Can you work these out from the model? Positions are in its coordinate system, mm. A direction names the side the tool comes from. Give positions to 0.01 mm unless a question says otherwise; leave off trailing zeros. Write each loop counter-clockwise with the first axis right and the second up, starting at its lowest first coordinate (ties: lowest second). Pieces come first, ordered by that corner, then holes.
from build123d import *

# Parameters (mm, degrees)
F1_DEPTH = 25.4


with BuildPart() as f1:
    # F0 (on Front) → F1 (new body)
    with BuildSketch(Plane.XZ):
        with BuildLine():
            Line((-1.5875, 51.919649), (-1.5875, 53.951649))
            ThreePointArc((-1.5875, 53.951649), (-9.37266, 53.154998), (-16.960789, 51.240924))
            Line((-16.960789, 51.240924), (-16.265804, 49.331468))
            Line((-16.265804, 49.331468), (-19.249328, 48.245554))
            Line((-19.249328, 48.245554), (-19.944313, 50.15501))
            ThreePointArc((-19.944313, 50.15501), (-26.9875, 46.743721), (-33.463356, 42.349787))
            Line((-33.463356, 42.349787), (-32.157212, 40.793184))
            Line((-32.157212, 40.793184), (-34.589403, 38.752334))
            Line((-34.589403, 38.752334), (-35.895547, 40.308936))
            ThreePointArc((-35.895547, 40.308936), (-41.347249, 34.694461), (-45.929749, 28.35064))
            Line((-45.929749, 28.35064), (-44.169985, 27.33464))
            Line((-44.169985, 27.33464), (-45.757485, 24.585009))
            Line((-45.757485, 24.585009), (-47.517249, 25.601009))
            ThreePointArc((-47.517249, 25.601009), (-50.719909, 18.460537), (-52.856336, 10.931988))
            Line((-52.856336, 10.931988), (-50.855207, 10.579135))
            Line((-50.855207, 10.579135), (-51.40654, 7.45237))
            Line((-51.40654, 7.45237), (-53.407669, 7.805223))
            ThreePointArc((-53.407669, 7.805223), (-53.975, 0), (-53.407669, -7.805223))
            Line((-53.407669, -7.805223), (-51.40654, -7.45237))
            Line((-51.40654, -7.45237), (-50.855207, -10.579135))
            Line((-50.855207, -10.579135), (-52.856336, -10.931988))
            ThreePointArc((-52.856336, -10.931988), (-50.719909, -18.460537), (-47.517249, -25.601009))
            Line((-47.517249, -25.601009), (-45.757485, -24.585009))
            Line((-45.757485, -24.585009), (-44.169985, -27.33464))
            Line((-44.169985, -27.33464), (-45.929749, -28.35064))
            ThreePointArc((-45.929749, -28.35064), (-41.347249, -34.694461), (-35.895547, -40.308936))
            Line((-35.895547, -40.308936), (-34.589403, -38.752334))
            Line((-34.589403, -38.752334), (-32.157212, -40.793184))
            Line((-32.157212, -40.793184), (-33.463356, -42.349787))
            ThreePointArc((-33.463356, -42.349787), (-26.9875, -46.743721), (-19.944313, -50.15501))
            Line((-19.944313, -50.15501), (-19.249328, -48.245554))
            Line((-19.249328, -48.245554), (-16.265804, -49.331468))
            Line((-16.265804, -49.331468), (-16.960789, -51.240924))
            ThreePointArc((-16.960789, -51.240924), (-9.37266, -53.154998), (-1.5875, -53.951649))
            Line((-1.5875, -53.951649), (-1.5875, -51.919649))
            Line((-1.5875, -51.919649), (1.5875, -51.919649))
            Line((1.5875, -51.919649), (1.5875, -53.951649))
            ThreePointArc((1.5875, -53.951649), (9.37266, -53.154998), (16.960789, -51.240924))
            Line((16.960789, -51.240924), (16.265804, -49.331468))
            Line((16.265804, -49.331468), (19.249328, -48.245554))
            Line((19.249328, -48.245554), (19.944313, -50.15501))
            ThreePointArc((19.944313, -50.15501), (26.9875, -46.743721), (33.463356, -42.349787))
            Line((33.463356, -42.349787), (32.157212, -40.793184))
            Line((32.157212, -40.793184), (34.589403, -38.752334))
            Line((34.589403, -38.752334), (35.895547, -40.308936))
            ThreePointArc((35.895547, -40.308936), (41.347249, -34.694461), (45.929749, -28.35064))
            Line((45.929749, -28.35064), (44.169985, -27.33464))
            Line((44.169985, -27.33464), (45.757485, -24.585009))
            Line((45.757485, -24.585009), (47.517249, -25.601009))
            ThreePointArc((47.517249, -25.601009), (50.719909, -18.460537), (52.856336, -10.931988))
            Line((52.856336, -10.931988), (50.855207, -10.579135))
            Line((50.855207, -10.579135), (51.40654, -7.45237))
            Line((51.40654, -7.45237), (53.407669, -7.805223))
            ThreePointArc((53.407669, -7.805223), (53.975, 0), (53.407669, 7.805223))
            Line((53.407669, 7.805223), (51.40654, 7.45237))
            Line((51.40654, 7.45237), (50.855207, 10.579135))
            Line((50.855207, 10.579135), (52.856336, 10.931988))
            ThreePointArc((52.856336, 10.931988), (50.719909, 18.460537), (47.517249, 25.601009))
            Line((47.517249, 25.601009), (45.757485, 24.585009))
            Line((45.757485, 24.585009), (44.169985, 27.33464))
            Line((44.169985, 27.33464), (45.929749, 28.35064))
            ThreePointArc((45.929749, 28.35064), (41.347249, 34.694461), (35.895547, 40.308936))
            Line((35.895547, 40.308936), (34.589403, 38.752334))
            Line((34.589403, 38.752334), (32.157212, 40.793184))
            Line((32.157212, 40.793184), (33.463356, 42.349787))
            ThreePointArc((33.463356, 42.349787), (26.9875, 46.743721), (19.944313, 50.15501))
            Line((19.944313, 50.15501), (19.249328, 48.245554))
            Line((19.249328, 48.245554), (16.265804, 49.331468))
            Line((16.265804, 49.331468), (16.960789, 51.240924))
            ThreePointArc((16.960789, 51.240924), (9.37266, 53.154998), (1.5875, 53.951649))
            Line((1.5875, 53.951649), (1.5875, 51.919649))
            Line((1.5875, 51.919649), (-1.5875, 51.919649))
        make_face()
        with BuildLine():
            ThreePointArc((-48.256028, -15.874375), (-50.028234, -8.821327), (-50.775189, -1.5875))
            Line((-50.775189, -1.5875), (-52.807189, -1.5875))
            Line((-52.807189, -1.5875), (-52.807189, 1.5875))
            Line((-52.807189, 1.5875), (-50.775189, 1.5875))
            ThreePointArc((-50.775189, 1.5875), (-50.028234, 8.821327), (-48.256028, 15.874375))
            Line((-48.256028, 15.874375), (-50.165483, 16.56936))
            Line((-50.165483, 16.56936), (-49.079569, 19.552884))
            Line((-49.079569, 19.552884), (-47.170114, 18.8579))
            ThreePointArc((-47.170114, 18.8579), (-43.994091, 25.4), (-39.916477, 31.421567))
            Line((-39.916477, 31.421567), (-41.473079, 32.727711))
            Line((-41.473079, 32.727711), (-39.432229, 35.159903))
            Line((-39.432229, 35.159903), (-37.875626, 33.853758))
            ThreePointArc((-37.875626, 33.853758), (-32.653611, 38.915058), (-26.76241, 43.178854))
            Line((-26.76241, 43.178854), (-27.77841, 44.938617))
            Line((-27.77841, 44.938617), (-25.028779, 46.526117))
            Line((-25.028779, 46.526117), (-24.012779, 44.766354))
            ThreePointArc((-24.012779, 44.766354), (-17.374623, 47.736385), (-10.380401, 49.728134))
            Line((-10.380401, 49.728134), (-10.733254, 51.729263))
            Line((-10.733254, 51.729263), (-7.60649, 52.280596))
            Line((-7.60649, 52.280596), (-7.253637, 50.279467))
            ThreePointArc((-7.253637, 50.279467), (0, 50.8), (7.253637, 50.279467))
            Line((7.253637, 50.279467), (7.60649, 52.280596))
            Line((7.60649, 52.280596), (10.733254, 51.729263))
            Line((10.733254, 51.729263), (10.380401, 49.728134))
            ThreePointArc((10.380401, 49.728134), (17.374623, 47.736385), (24.012779, 44.766354))
            Line((24.012779, 44.766354), (25.028779, 46.526117))
            Line((25.028779, 46.526117), (27.77841, 44.938617))
            Line((27.77841, 44.938617), (26.76241, 43.178854))
            ThreePointArc((26.76241, 43.178854), (32.653611, 38.915058), (37.875626, 33.853758))
            Line((37.875626, 33.853758), (39.432229, 35.159903))
            Line((39.432229, 35.159903), (41.473079, 32.727711))
            Line((41.473079, 32.727711), (39.916477, 31.421567))
            ThreePointArc((39.916477, 31.421567), (43.994091, 25.4), (47.170114, 18.8579))
            Line((47.170114, 18.8579), (49.079569, 19.552884))
            Line((49.079569, 19.552884), (50.165483, 16.56936))
            Line((50.165483, 16.56936), (48.256028, 15.874375))
            ThreePointArc((48.256028, 15.874375), (50.028234, 8.821327), (50.775189, 1.5875))
            Line((50.775189, 1.5875), (52.807189, 1.5875))
            Line((52.807189, 1.5875), (52.807189, -1.5875))
            Line((52.807189, -1.5875), (50.775189, -1.5875))
            ThreePointArc((50.775189, -1.5875), (50.028234, -8.821327), (48.256028, -15.874375))
            Line((48.256028, -15.874375), (50.165483, -16.56936))
            Line((50.165483, -16.56936), (49.079569, -19.552884))
            Line((49.079569, -19.552884), (47.170114, -18.8579))
            ThreePointArc((47.170114, -18.8579), (43.994091, -25.4), (39.916477, -31.421567))
            Line((39.916477, -31.421567), (41.473079, -32.727711))
            Line((41.473079, -32.727711), (39.432229, -35.159903))
            Line((39.432229, -35.159903), (37.875626, -33.853758))
            ThreePointArc((37.875626, -33.853758), (32.653611, -38.915058), (26.76241, -43.178854))
            Line((26.76241, -43.178854), (27.77841, -44.938617))
            Line((27.77841, -44.938617), (25.028779, -46.526117))
            Line((25.028779, -46.526117), (24.012779, -44.766354))
            ThreePointArc((24.012779, -44.766354), (17.374623, -47.736385), (10.380401, -49.728134))
            Line((10.380401, -49.728134), (10.733254, -51.729263))
            Line((10.733254, -51.729263), (7.60649, -52.280596))
            Line((7.60649, -52.280596), (7.253637, -50.279467))
            ThreePointArc((7.253637, -50.279467), (0, -50.8), (-7.253637, -50.279467))
            Line((-7.253637, -50.279467), (-7.60649, -52.280596))
            Line((-7.60649, -52.280596), (-10.733254, -51.729263))
            Line((-10.733254, -51.729263), (-10.380401, -49.728134))
            ThreePointArc((-10.380401, -49.728134), (-17.374623, -47.736385), (-24.012779, -44.766354))
            Line((-24.012779, -44.766354), (-25.028779, -46.526117))
            Line((-25.028779, -46.526117), (-27.77841, -44.938617))
            Line((-27.77841, -44.938617), (-26.76241, -43.178854))
            ThreePointArc((-26.76241, -43.178854), (-32.653611, -38.915058), (-37.875626, -33.853758))
            Line((-37.875626, -33.853758), (-39.432229, -35.159903))
            Line((-39.432229, -35.159903), (-41.473079, -32.727711))
            Line((-41.473079, -32.727711), (-39.916477, -31.421567))
            ThreePointArc((-39.916477, -31.421567), (-43.994091, -25.4), (-47.170114, -18.8579))
            Line((-47.170114, -18.8579), (-49.079569, -19.552884))
            Line((-49.079569, -19.552884), (-50.165483, -16.56936))
            Line((-50.165483, -16.56936), (-48.256028, -15.874375))
        make_face(mode=Mode.SUBTRACT)
    extrude(amount=F1_DEPTH)


solid = f1.part
(1) If we mould it in two halves opening along X, with no side actions, what happens to faces 4 (the face through (17.47, -12.52, -47.7)), 5 (the face through (26.89, -12.52, -46.8)), 6 (the face through (-32, -25.4, -40))? For each: +X half, -X half, draft (parallel to the pull), parting line (faces both ways), or undercut.
Returned:
face 4: undercut
face 5: +X half
face 6: draft
(2) Will these pins go through, and if not, where does the flat tip stop? P1, Ø3.5, axis at x = 0.5, y = -11.5, coming from the +Z side; P2, Ø12, axis at y = -16, z = 31.5, coming from the +X side; P3, Ø1, axis at y = -4.5, z = 31, coming from the +X side; P4, Ø1, axis at x = -0.5, y = -16.5, coming from the -Z side.
Returned:
P1: stops at z = 53.95
P2: stops at x = 47.57
P3: stops at x = 44.53
P4: stops at z = -51.92
(3) Imagine slicing it at B-B, the plane x = 30. Write out the boundary of the cut face in (y, z).
Returned:
outline: (-25.4, -44.87) - (0, -44.87) - (0, -41) - (-25.4, -41) - close; (-25.4, 41) - (0, 41) - (0, 44.87) - (-25.4, 44.87) - close
(4) Imagine slicing it at A-A, the plane x = 13. Write out the boundary of the cut face in (y, z).
Returned:
outline: (-25.4, -52.39) - (0, -52.39) - (0, -49.11) - (-25.4, -49.11) - close; (-25.4, 49.11) - (0, 49.11) - (0, 52.39) - (-25.4, 52.39) - close
(5) For faces 1 (the face through (17.78, -12.52, 48.78)), 2 (the face through (0, -13, -51.92)), 3 (the face through (-9.481, -12.522, -53.136)), which set-ups out of +Z, -Z, +X, -X, +Y, -Y let a thin tool reach every point of the face, with its end or its side?
Returned:
face 1: +Y, -Y
face 2: -Z, +Y, -Y
face 3: -Z, -X, +Y, -Y
(6) If I drill on L1, parallel to Z at x = 33, y = -6.5; L2, parallel to X at y = -9.75, z = -10.5; L3, parallel to Z at x = 27.5, y = -2.75, over which ranges is the centre line in solid material (lowest first)?
Returned:
L1: z = -42.71 to -41.8, -40.09 to -38.62, 38.62 to 40.09, 41.8 to 42.71
L2: x = -50.87 to -49.7, 49.7 to 50.87
L3: z = -46.44 to -45.1, -44.46 to -42.71, 42.71 to 44.46, 45.1 to 46.44
